For this review, take the finished solid that the model builds, in its own axes (mm). Face numbers are marked on the shaded views. A direction names the side the tool comes from. Give positions to 0.01 mm unless a question says otherwise; leave off trailing zeros. Write each loop counter-clockwise with the first axis right and the second up, starting at its lowest first coordinate (ties: lowest second). Pieces come first, ordered by that corner, then holes. Notation, with made-up numbers: M -29,3.25 L -19,3.25 A11 ccw -19,24.25 Z; hole C 15.5,-16 d11. An arc over 180 degrees is marked long. Write item = value, one per line.
```python
from build123d import *

# Parameters (mm, degrees)
SKETCH1_R               = 17.75
SKETCH1_R_2             = 15
BOSS_EXTRUDE1_DEPTH     = 45
SKETCH2_W               = 16.5
SKETCH2_H               = 11.5
CUT_EXTRUDE1_DEPTH      = 2.5
CUT_EXTRUDE2_REACH      = 60.726
CUT_EXTRUDE2_END_RADIUS = 15
SKETCH3_R               = 4.5
CIRPATTERN1_COUNT       = 2
CIRPATTERN1_ANGLE       = 90


with BuildPart() as part:
    # Sketch1 → Boss-Extrude1 (new body)
    with BuildSketch(Plane(origin=(0, 0, 0), x_dir=(1, 0, 0), z_dir=(0, 1, 0))):
        with Locations(Location((0, 0.545038043, 0), (0, 0, 90))):
            Circle(SKETCH1_R)
        with Locations(Location((0, 0.545038043, 0), (0, 0, 90))):
            Circle(SKETCH1_R_2, mode=Mode.SUBTRACT)
    extrude(amount=BOSS_EXTRUDE1_DEPTH)

    # Sketch2 → Cut-Extrude1 (cut)
    with BuildSketch(Plane(origin=(17.75, 0, 0), x_dir=(0, 0, -1), z_dir=(1, 0, 0))):
        with Locations((0, 8.243102377)):
            Rectangle(SKETCH2_W, SKETCH2_H)
    cut_extrude1 = extrude(amount=-CUT_EXTRUDE1_DEPTH, mode=Mode.SUBTRACT)

    # Cut-Extrude2: up to this cylinder (the profile starts outside it)
    cut_extrude2_end = Plane(origin=(0, 8.243102, -0.545038043), z_dir=(0, -1, 0)) * Cylinder(CUT_EXTRUDE2_END_RADIUS, 152.452, mode=Mode.PRIVATE)
    # Sketch3 → Cut-Extrude2 (cut, up to the surface)
    with BuildSketch(Plane(origin=(15.25, 0, 0), x_dir=(0, 0, -1), z_dir=(1, 0, 0)), mode=Mode.PRIVATE) as cut_extrude2_sk1:
        with Locations((-0.25, 8.243102377)):
            Circle(SKETCH3_R)
    cut_extrude2_tool1 = extrude(cut_extrude2_sk1.sketch, amount=-CUT_EXTRUDE2_REACH, mode=Mode.PRIVATE) - cut_extrude2_end
    cut_extrude2 = cut_extrude2_tool1.solids().sort_by_distance((15.25, 8.243102, 0.25))[0]
    add(cut_extrude2, mode=Mode.SUBTRACT)

    # CirPattern1: Cut-Extrude1, Cut-Extrude2 ×2 about axis
    cirpattern1_axis = Axis((0, 0, -0.545038043), (0, 1, 0))
    add([cut_extrude1.rotate(cirpattern1_axis, i * CIRPATTERN1_ANGLE / (CIRPATTERN1_COUNT - 1)) for i in range(1, CIRPATTERN1_COUNT)], mode=Mode.SUBTRACT)
    add([cut_extrude2.rotate(cirpattern1_axis, i * CIRPATTERN1_ANGLE / (CIRPATTERN1_COUNT - 1)) for i in range(1, CIRPATTERN1_COUNT)], mode=Mode.SUBTRACT)


solid = part.part
```
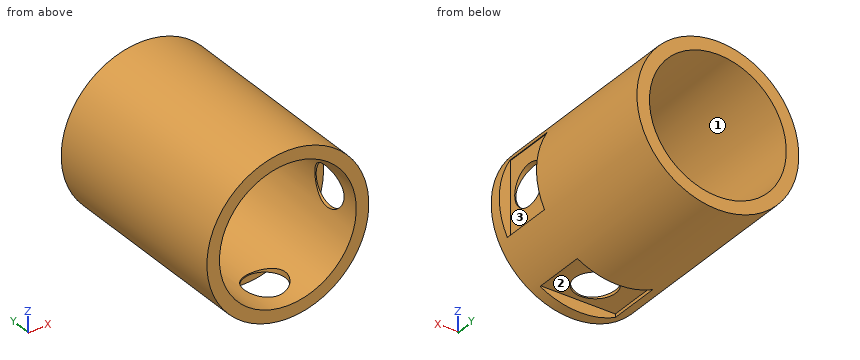
1. We need section B-B, the plane z = 9.5. Write out the cut boundary in (x, y).
Responses:
outline = M -14.63,0 L -11.14,0 L -11.14,45 L -14.63,45 Z; M 11.14,0 L 14.63,0 L 14.63,45 L 11.14,45 Z
2. Machinability: for the marked faces 1, 2 and 3, which of the approach directions +Z, -Z, +X, -X, +Y, -Y give a long, thin tool a straight path to every point of the face, cutting with its end or side? Answer none if there is none.
Responses:
face_1 = +Y, -Y
face_2 = -Z
face_3 = +X
3. We need section A-A, the plane x = 10.5. Write out the cut boundary in (y, z), then the cut area to 3 significant figures.
Responses:
outline = M 0,-14.86 L 45,-14.86 L 45,-11.26 L 0,-11.26 Z; M 0,10.17 L 45,10.17 L 45,13.77 L 0,13.77 Z
area = 324 mm2
4. For line 1 along Y through (x, z) = (3, -17); line 2 along Z through (x, y) = (13.5, 15); line 3 along X through (y, z) = (37, -5), list the stretches that pass through material, from the lowest coordinate up. Write a range as from..to.
Responses:
line_1 = 0..2.49, 13.99..45
line_2 = -12.07..-7.08, 5.99..10.98
line_3 = -17.18..-14.32, 14.32..17.18
5. We need section C-C, the plane x = 0. Write out the cut boundary in (y, z).
Responses:
outline = M 0,-18.3 L 2.49,-18.3 L 2.49,-15.8 L 3.81,-15.8 L 3.81,-15.55 L 0,-15.55 Z; M 0,14.45 L 45,14.45 L 45,17.2 L 0,17.2 Z; M 12.67,-15.8 L 13.99,-15.8 L 13.99,-18.3 L 45,-18.3 L 45,-15.55 L 12.67,-15.55 Z
6. We need section D-D, the plane y = 17.5. Write out the cut boundary in (x, z), then the cut area to 3 significant figures.
Responses:
outline = C 0,-0.55 d35.5; hole C 0,-0.55 d30
area = 283 mm2
7. Insertion check: P1, Ø8, axis at x = 1.5, y = 26.5, coming from the +Z side; P2, Ø3, axis at y = 30, z = -10, coming from the -X side; P3, Ø5, axis at y = 9, z = 12.5, coming from the +X side; P4, Ø8, axis at y = 13.5, z = 11, coming from the -X side. Each pin has a flat end and moves straight along its axis. Give the tip position at first contact, or say it passes through.
Responses:
P1 = 17.2
P2 = -15.87
P3 = 14.28
P4 = -16.07
